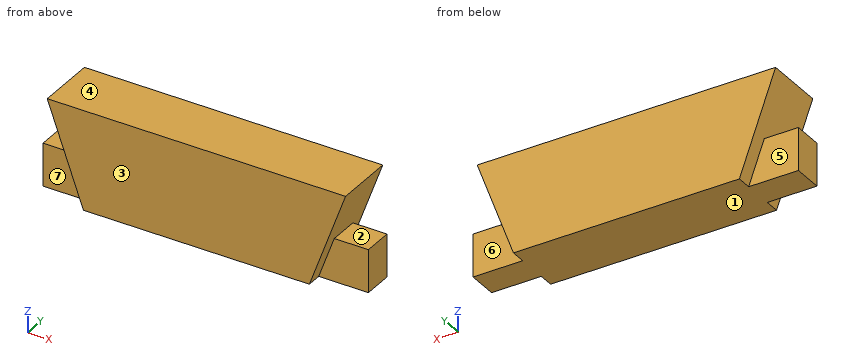
```python
from build123d import *

# Parameters (mm, degrees)
SALIENTE_EXTRUIR4_DEPTH = 30
CROQUIS6_W              = 163.6
CROQUIS6_H              = 15
SALIENTE_EXTRUIR6_DEPTH = 21.55


with BuildPart() as part:
    # Croquis3 → Saliente-Extruir4 (new body)
    with BuildSketch(Plane(origin=(0, 0, 0), x_dir=(1, 0, 0), z_dir=(0, 1, 0))):
        Polygon((-75, 0), (75, 0), (56.801488287, 50), (-56.801488287, 50), align=None)
    extrude(amount=SALIENTE_EXTRUIR4_DEPTH)

    # Croquis6 → Saliente-Extruir6 (add)
    with BuildSketch(Plane(origin=(0, 0, -50), x_dir=(-1, 0, 0), z_dir=(0, 0, -1))):
        with Locations((0, 15)):
            Rectangle(CROQUIS6_W, CROQUIS6_H)
    extrude(amount=-SALIENTE_EXTRUIR6_DEPTH)


solid = part.part
```
Part model, mm, in its own coordinate system. Face numbers are marked on the shaded views. A direction names the side the tool comes from. Round coordinates to 2 decimals unless told otherwise and drop trailing zeros. Order: outer loops, then holes, each group sorted by start corner. A loop starts at its lowest first (then second) coordinate and runs counter-clockwise, first axis right, second up. Notation, with made-up numbers: M 4.25,-21.5 L 57.25,-21.5 A19 ccw 57.25,15.5 Z; hole C -3.5,-25.5 d7. An arc over 180 degrees is marked long. Answer in a Markdown table with one row per item. Add a question column.
Q1. Wall check: L1, parallel to Y at x = -74, z = -43; L2, parallel to X at y = 5.5, z = -7; L3, parallel to X at y = 17.5, z = -15. Give the ranges that are in metal, low to high. Write a range as from..to.
Q2. Cut at A-A on y = 18.25. Give the cut face in (x, z), and give its area (3 significant figures).
Q3. Cut at D-D on z = -33.5. Give the cut face in (x, y), and give its area (3 significant figures).
Q4. 3-axis set-ups, long thin cutter, end or side, ignore diameter. For the marked faces 5, 6 and 7: which of +Z, -Z, +X, -X, +Y, -Y reach the whole face in a straight line?
Q5. Mould opens along Z. For the marked faces 1, 2, 3 and 4 say: +Z half, -Z half, draft (parallel to the pull), parting line (faces both ways), or undercut.
Q6. Cut at B-B on z = -45. Give the cut face in (x, y), and give its area (3 significant figures).
Q7. Cut at C-C on x = -62. Give the cut face in (y, z).
Q8. Pin check, flat tips, straight feed: pin 1 (6.5 mm diameter, centred on x = 73, z = -44, fed in from -Y); pin 2 (1 mm diameter, centred on y = 13.5, z = -21, fed in from -X); pin 3 (5 mm diameter, centred on y = 8.5, z = -19, fed in from +X). Stop position of each tip, or through.
Established:
| question | item | result |
|---|---|---|
| 1 | L1 | y = 7.5..22.5 |
| 1 | L2 | x = -72.45..72.45 |
| 1 | L3 | x = -69.54..69.54 |
| 2 | outline | M -81.8,-50 L 81.8,-50 L 81.8,-28.45 L 64.65,-28.45 L 75,0 L -75,0 L -64.65,-28.45 L -81.8,-28.45 Z |
| 2 | area | 7,500 mm2 |
| 3 | outline | M -81.8,7.5 L -62.81,7.5 L -62.81,0 L 62.81,0 L 62.81,7.5 L 81.8,7.5 L 81.8,22.5 L 62.81,22.5 L 62.81,30 L -62.81,30 L -62.81,22.5 L -81.8,22.5 Z |
| 3 | area | 4,340 mm2 |
| 4 | face 5 | -Z, -X, +Y |
| 4 | face 6 | -Z, +X, +Y |
| 4 | face 7 | -Z, -X, -Y |
| 5 | face 1 | -Z half |
| 5 | face 2 | undercut |
| 5 | face 3 | draft |
| 5 | face 4 | +Z half |
| 6 | outline | M -81.8,7.5 L -58.62,7.5 L -58.62,0 L 58.62,0 L 58.62,7.5 L 81.8,7.5 L 81.8,22.5 L 58.62,22.5 L 58.62,30 L -58.62,30 L -58.62,22.5 L -81.8,22.5 Z |
| 6 | area | 4,210 mm2 |
| 7 | outline | M 0,-35.72 L 7.5,-35.72 L 7.5,-50 L 22.5,-50 L 22.5,-35.72 L 30,-35.72 L 30,0 L 0,0 Z |
| 8 | pin 1 | stops at y = 7.5 |
| 8 | pin 2 | stops at x = -67.54 |
| 8 | pin 3 | stops at x = 68.99 |
